Geometry: final body of the model. Coordinates: model frame, mm. Round coordinates to 2 decimals unless told otherwise and drop trailing zeros. Loops run counter-clockwise (first coordinate to the right, second up) from the corner with the lowest first, then second, coordinate; pieces in that order, holes last. Notation, with made-up numbers: (68, -19) - (95, -19) arc R10 ccw to (95, -14) - close; hole circle Ø5 at (-8, 84.5). An arc over 180 degrees is marked (long way). Answer as a JSON object with one key per item and string values. Group by question number.
Item 1: Draft query along X for faces 1 (the face through (0.285, 6.699, 2.958)), 2 (the face through (7, 5, 0)), 3 (the face through (2.77, 3.45, 5.15)). Return one class per face: released by +X, released by -X, zero draft, split by the parting line, or undercut.
Item 2: Line query: line 1 (Y direction, x = 6, z = 2.35); line 2 (X direction, y = 1.75, z = 5.45); line 3 (Y direction, x = 5.25, z = 3.2). Output: solid intervals per line, ascending.
Item 3: Section A-A (z = 3.25). Return the cut outline in (x, y).
Item 4: Section B-B (x = 6). Return the cut outline in (y, z), plus the area to 3 significant figures.
Item 5: Section C-C (y = 3.5). Return the cut outline in (x, z).
Item 6: Section D-D (y = 6.75). Return the cut outline in (x, z).
```python
from build123d import *

# Parameters (mm, degrees)
SKETCH1_R           = 1.6
BOSS_EXTRUDE1_DEPTH = 6
CUT_EXTRUDE1_DEPTH  = 7


with BuildPart() as part:
    # Sketch1 → Boss-Extrude1 (new body)
    with BuildSketch(Plane.XY):
        with BuildLine():
            Line((12, 6), (12, 1))
            ThreePointArc((12, 1), (11.707106781, 0.292893219), (11, 0))
            Line((11, 0), (1, 0))
            ThreePointArc((1, 0), (0.292893219, 0.292893219), (0, 1))
            Line((0, 1), (0, 6))
            ThreePointArc((0, 6), (0.292893219, 6.707106781), (1, 7))
            Line((1, 7), (11, 7))
            ThreePointArc((11, 7), (11.707106781, 6.707106781), (12, 6))
        make_face()
        with Locations((6, 3.5)):
            Circle(SKETCH1_R, mode=Mode.SUBTRACT)
    extrude(amount=BOSS_EXTRUDE1_DEPTH)

    # Sketch2 → Cut-Extrude1 (cut)
    with BuildSketch(Plane.XZ):
        with BuildLine():
            Line((1.9, 6), (3.6, 6))
            ThreePointArc((3.6, 6), (2.75, 5.15), (1.9, 6))
        make_face()
        with BuildLine():
            Line((8.4, 6), (10.1, 6))
            ThreePointArc((10.1, 6), (9.25, 5.15), (8.4, 6))
        make_face()
    extrude(amount=-CUT_EXTRUDE1_DEPTH, mode=Mode.SUBTRACT)


solid = part.part
```
Values:
{
 "1": {"face 1": "released by -X", "face 2": "zero draft", "face 3": "undercut"},
 "2": {"line 1": "y = 0 to 1.9, 5.1 to 7", "line 2": "x = 0 to 2.1, 3.4 to 8.6, 9.9 to 12", "line 3": "y = 0 to 2.09, 4.91 to 7"},
 "3": {"outline": "(0, 1) arc R1 ccw to (1, 0) - (11, 0) arc R1 ccw to (12, 1) - (12, 6) arc R1 ccw to (11, 7) - (1, 7) arc R1 ccw to (0, 6) - close; hole circle Ø3.2 at (6, 3.5)"},
 "4": {"outline": "(0, 0) - (1.9, 0) - (1.9, 6) - (0, 6) - close; (5.1, 0) - (7, 0) - (7, 6) - (5.1, 6) - close", "area": "22.8 mm^2"},
 "5": {"outline": "(0, 0) - (4.4, 0) - (4.4, 6) - (3.6, 6) arc R0.85 cw to (1.9, 6) - (0, 6) - close; (7.6, 0) - (12, 0) - (12, 6) - (10.1, 6) arc R0.85 cw to (8.4, 6) - (7.6, 6) - close"},
 "6": {"outline": "(0.34, 0) - (11.66, 0) - (11.66, 6) - (10.1, 6) arc R0.85 cw to (8.4, 6) - (3.6, 6) arc R0.85 cw to (1.9, 6) - (0.34, 6) - close"}
}
